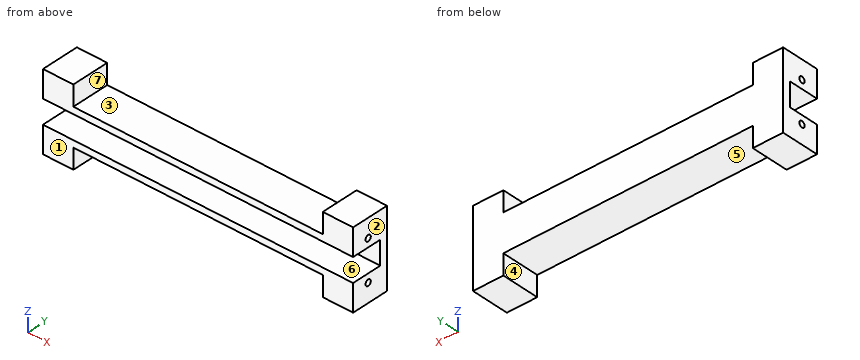
```python
from build123d import *

# Parameters (mm, degrees)
SKETCH1_W           = 183.96444
SKETCH1_H           = 22
BOSS_EXTRUDE1_DEPTH = 22.5
SKETCH2_W           = 183.96444
SKETCH2_H           = 14
CUT_EXTRUDE1_DEPTH  = 18
SKETCH3_W           = 18
SKETCH3_H           = 22.5
BOSS_EXTRUDE2_DEPTH = 12
SKETCH4_W           = 18
SKETCH4_H           = 22.5
BOSS_EXTRUDE3_DEPTH = 12
SKETCH5_R           = 1.7526
CUT_EXTRUDE2_DEPTH  = 16
CUT_EXTRUDE3_START  = -16
SKETCH6_R           = 1.7526
CUT_EXTRUDE3_DEPTH  = 16


with BuildPart() as part:
    # Sketch1 → Boss-Extrude1 (new body)
    with BuildSketch(Plane(origin=(0, 0, 0), x_dir=(1, 0, 0), z_dir=(0, 1, 0))):
        Rectangle(SKETCH1_W, SKETCH1_H)
    extrude(amount=BOSS_EXTRUDE1_DEPTH)

    # Sketch2 → Cut-Extrude1 (cut)
    with BuildSketch(Plane.XZ):
        Rectangle(SKETCH2_W, SKETCH2_H)
    extrude(amount=-CUT_EXTRUDE1_DEPTH, mode=Mode.SUBTRACT)

    # Sketch3 → Boss-Extrude2 (add)
    with BuildSketch(Plane.XY.offset(11)):
        with Locations((-82.98222, 11.25)):
            Rectangle(SKETCH3_W, SKETCH3_H)
        with Locations((82.98222, 11.25)):
            Rectangle(SKETCH3_W, SKETCH3_H)
    extrude(amount=BOSS_EXTRUDE2_DEPTH)

    # Sketch4 → Boss-Extrude3 (add)
    with BuildSketch(Plane(origin=(0, 0, -11), x_dir=(-1, 0, 0), z_dir=(0, 0, -1))):
        with Locations((-82.98222, 11.25)):
            Rectangle(SKETCH4_W, SKETCH4_H)
        with Locations((82.98222, 11.25)):
            Rectangle(SKETCH4_W, SKETCH4_H)
    extrude(amount=BOSS_EXTRUDE3_DEPTH)

    # Sketch5 → Cut-Extrude2 (cut)
    with BuildSketch(Plane(origin=(91.98222, 0, 0), x_dir=(0, 0, -1), z_dir=(1, 0, 0))):
        with Locations((-12, 10)):
            Circle(SKETCH5_R)
        with Locations((12, 10)):
            Circle(SKETCH5_R)
    extrude(amount=-CUT_EXTRUDE2_DEPTH, mode=Mode.SUBTRACT)

    # Sketch6 → Cut-Extrude3 (cut)
    with BuildSketch(Plane.ZY.offset(91.98222).offset(CUT_EXTRUDE3_START)):
        with Locations(Location((-12, 10, 0), (0, 0, 180))):
            Circle(SKETCH6_R)
        with Locations(Location((12, 10, 0), (0, 0, 180))):
            Circle(SKETCH6_R)
    extrude(amount=CUT_EXTRUDE3_DEPTH, mode=Mode.SUBTRACT)


solid = part.part
```
The listing builds one solid part. Answer for the finished solid, in the listing's coordinates (mm). Face numbers are marked on the shaded views. A direction names the side the tool comes from. Give positions to 0.01 mm unless a question says otherwise; leave off trailing zeros. Order: outer loops, then holes, each group sorted by start corner. A loop starts at its lowest first (then second) coordinate and runs counter-clockwise, first axis right, second up. Notation, with made-up numbers: (64, -36.5) -> (121, -36.5) arc R18 ccw to (121, -25.5) -> close; hole circle Ø1 at (-39, 29). An arc over 180 degrees is marked (long way). Answer as a JSON object with one key per item and string values. Group by question number.
Item 1: A tool of negligible diameter and unlimited length cuts with its end or side. For the marked faces 5, 6 and 7, from which of +Z, -Z, +X, -X, +Y, -Y can it reach the whole face along a straight path? Write none if from no direction.
Item 2: The part is cut by section C-C on y = 3. Write down the section's boundary in (x, z).
Item 3: The part is cut by section D-D on z = -1.5. Write down the section's boundary in (x, y), and give its area (3 significant figures).
Item 4: Consider L1, parallel to Z at x = -81.5, y = 10; L2, parallel to X at y = 15.75, z = -18.5; L3, parallel to Z at x = 29, y = 2. Determine where each line is inside the solid, lowest interval first. Write a range as from..to.
Item 5: Determine the mould class of the marked faces 1, 2, 3 and 4 for opening direction X: pulls with the +X half, pulls with the -X half, needs draft (parallel to the pull), parting line crosses it, or undercut.
Item 6: The part is cut by section B-B on x = -64.5. Write down the section's boundary in (y, z).
Item 7: Flat-ended cylindrical pins translate along their axes: pin 1 (1.8 mm diameter, centred on y = 10, z = -12.5, fed in from +X); pin 2 (9 mm diameter, centred on x = 23, y = 6.5, fed in from +Z); pin 3 (2 mm diameter, centred on x = -71.5, y = 17, fed in from -Z). Find the tip coordinate at first contact, or state that the pin passes through.
Result set:
{
 "1": {"face 5": "-Z, +Y, -Y", "face 6": "+X, -X, -Y", "face 7": "+Z, +Y, -Y"},
 "2": {"outline": "(-91.98, -23) -> (-73.98, -23) -> (-73.98, -11) -> (73.98, -11) -> (73.98, -23) -> (91.98, -23) -> (91.98, -7) -> (-91.98, -7) -> close; (-91.98, 7) -> (91.98, 7) -> (91.98, 23) -> (73.98, 23) -> (73.98, 11) -> (-73.98, 11) -> (-73.98, 23) -> (-91.98, 23) -> close"},
 "3": {"outline": "(-91.98, 18) -> (91.98, 18) -> (91.98, 22.5) -> (-91.98, 22.5) -> close", "area": "828 mm²"},
 "4": {"L1": "-23..-13.75, -10.25..-7, 7..10.25, 13.75..23", "L2": "-91.98..-73.98, 73.98..91.98", "L3": "-11..-7, 7..11"},
 "5": {"face 1": "needs draft", "face 2": "pulls with the +X half", "face 3": "undercut", "face 4": "undercut"},
 "6": {"outline": "(0, -11) -> (22.5, -11) -> (22.5, 11) -> (0, 11) -> (0, 7) -> (18, 7) -> (18, -7) -> (0, -7) -> close"},
 "7": {"pin 1": "x = 75.98", "pin 2": "z = 11", "pin 3": "z = -11"}
}
